Design review of the part shown in the three views and the two pictorial views. Dimensions are in mm from the part's minimum x, y and z. A direction names the side the tool comes from. Round coordinates to 2 decimals unless told otherwise and drop trailing zeros. Order: outer loops, then holes, each group sorted by start corner. A loop starts at its lowest first (then second) coordinate and runs counter-clockwise, first axis right, second up.
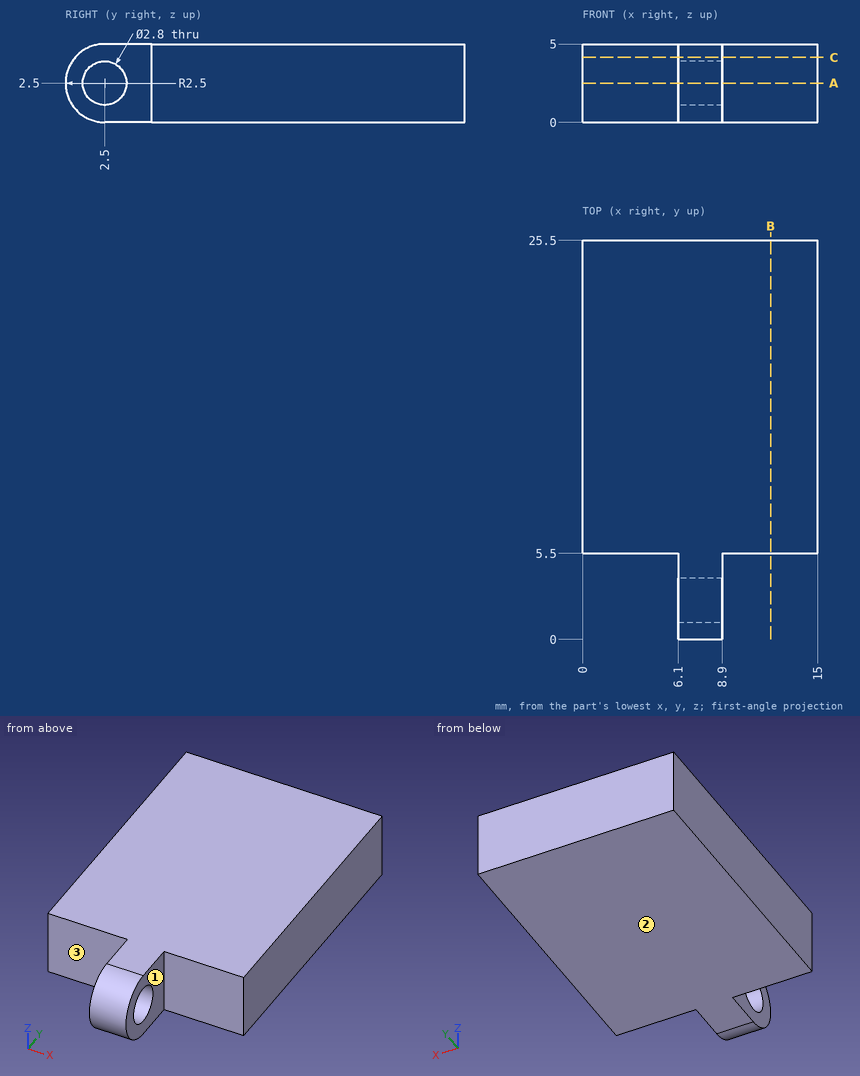
1) To check wall thickness, follow line 1 along Z through (x, y) = (7.9, 2.5); line 2 along Y through (x, z) = (6, 1.6); line 3 along X through (y, z) = (4.25, 4.75). State the ranges of each line that lie inside material, in increasing order.
Results:
line 1: z = 0 to 1.1, 3.9 to 5
line 2: y = 5.5 to 25.5
line 3: x = 6.1 to 8.9
2) Take a section at B-B on x = 12. Give the boundary of the cut face in (y, z).
Results:
outline: (5.5, 0) - (25.5, 0) - (25.5, 5) - (5.5, 5) - close
3) Take a section at A-A on z = 2.5. Give the boundary of the cut face in (x, y).
Results:
outline: (0, 5.5) - (6.1, 5.5) - (6.1, 3.9) - (8.9, 3.9) - (8.9, 5.5) - (15, 5.5) - (15, 25.5) - (0, 25.5) - close; (6.1, 0) - (8.9, 0) - (8.9, 1.1) - (6.1, 1.1) - close
4) Take a section at C-C on z = 4.15. Give the boundary of the cut face in (x, y).
Results:
outline: (0, 5.5) - (6.1, 5.5) - (6.1, 0.62) - (8.9, 0.62) - (8.9, 5.5) - (15, 5.5) - (15, 25.5) - (0, 25.5) - close
5) Clearance check with flat-ended pins moving along their axes: P1, Ø5, axis at x = 7.5, y = 21, coming from the -Z side; P2, Ø1.5, axis at y = 1.5, z = 3, coming from the +X side; P3, Ø3, axis at x = 3, z = 2, coming from the -Y side; P4, Ø2.5, axis at y = 2, z = 2.5, coming from the -X side. State where each tip first meets the part, or that it passes through.
Results:
P1: stops at z = 0
P2: stops at x = 8.9
P3: stops at y = 5.5
P4: stops at x = 6.1
6) For the marked faces 1, 2 and 3, list the 3-axis set-ups (+Z, -Z, +X, -X, +Y, -Y) from which the entire face can be reached by the end or side of a thin tool; tool diameter is ignored.
Results:
face 1: +Z, -Z, +X, -Y
face 2: -Z, +X, -X, +Y, -Y
face 3: +Z, -Z, -X, -Y
